Study the drawing (mm; zero at the part's minimum x, y, z) and answer. A direction names the side the tool comes from. Coordinates: 2 decimals unless noted, no trailing zeros. Order: outer loops, then holes, each group sorted by start corner. A loop starts at its lowest first (then second) coordinate and runs counter-clockwise, first axis right, second up.
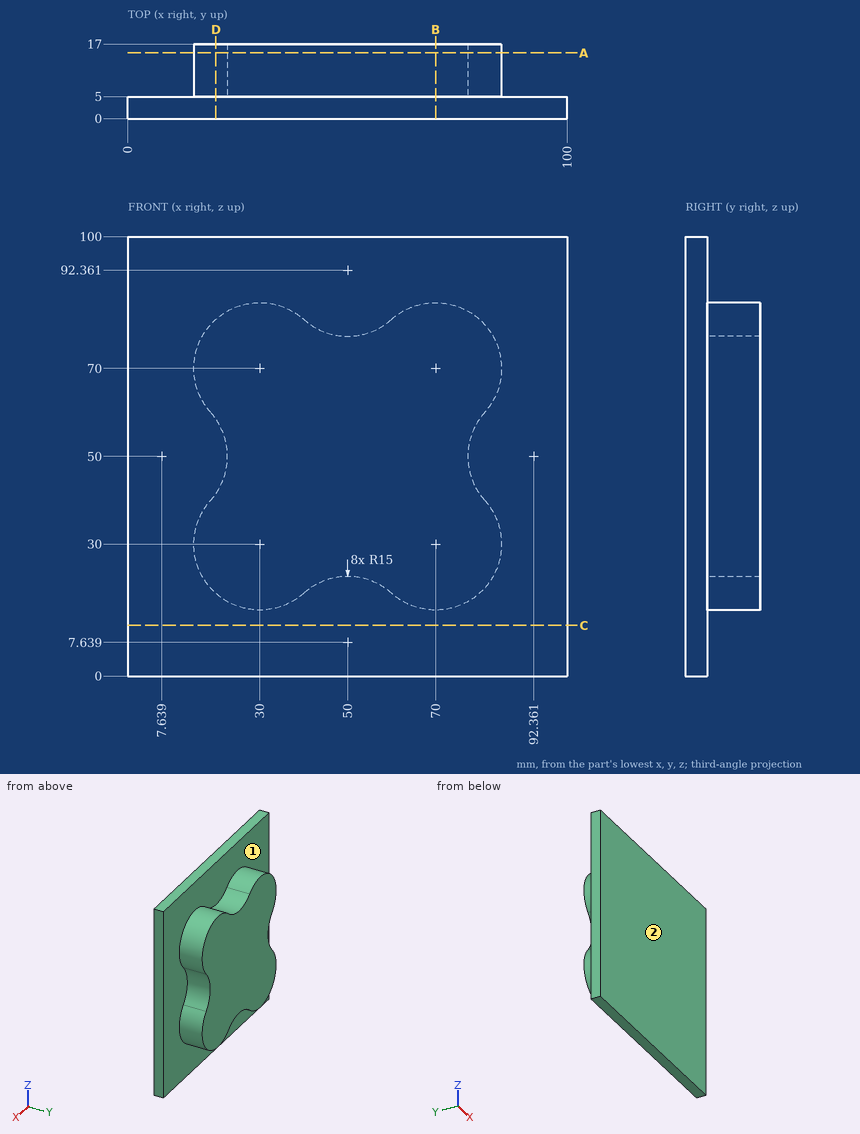
1) Straight lines are drawn through the part: line 1 (Y direction, x = 25, z = 94); line 2 (Z direction, x = 32.5, y = 13); line 3 (Z direction, x = 39, y = 14.5). For each, find the intervals that lie inside material, in ascending order.
A:
line 1: y = 0 to 5
line 2: z = 15.21 to 84.79
line 3: z = 18 to 82
2) A cutting plane is placed at D-D, the plane x = 20. Determine the outline of the cut face in (y, z), and give its area (3 significant figures).
A:
outline: (0, 0) - (5, 0) - (5, 18.82) - (17, 18.82) - (17, 41.5) - (5, 41.5) - (5, 58.5) - (17, 58.5) - (17, 81.18) - (5, 81.18) - (5, 100) - (0, 100) - close
area: 1,040 mm2
3) A cutting plane is placed at A-A, the plane y = 15. Determine the outline of the cut face in (x, z), and give its area (3 significant figures).
A:
outline: (18.82, 40) arc R15 ccw to (40, 18.82) arc R15 cw to (60, 18.82) arc R15 ccw to (81.18, 40) arc R15 cw to (81.18, 60) arc R15 ccw to (60, 81.18) arc R15 cw to (40, 81.18) arc R15 ccw to (18.82, 60) arc R15 cw to start
area: 4,100 mm2
4) Which of the six approach directions +Z, -Z, +X, -X, +Y, -Y give full straight-line access (tool end or side, diameter ignored) to the marked faces 1 and 2?
A:
face 1: +Y
face 2: +Z, -Z, +X, -X, -Y
5) A cutting plane is placed at C-C, the plane z = 11.5. Determine the outline of the cut face in (x, y).
A:
outline: (0, 0) - (100, 0) - (100, 5) - (0, 5) - close
6) A cutting plane is placed at B-B, the plane x = 70. Determine the outline of the cut face in (y, z), and give its area (3 significant figures).
A:
outline: (0, 0) - (5, 0) - (5, 15) - (17, 15) - (17, 85) - (5, 85) - (5, 100) - (0, 100) - close
area: 1,340 mm2
7) Flat-ended cylindrical pins translate along their axes: pin 1 Ø10 at (x, z) = (21.5, 69) entering from -Y; pin 2 Ø4 at (y, z) = (9.5, 28) entering from +X. Find the tip coordinate at first contact, or state that the pin passes through.
A:
pin 1: stops at y = 0
pin 2: stops at x = 85
